Work out the finished part from the listing and answer in its coordinate system (mm). Round coordinates to 2 decimals unless told otherwise and drop trailing zeros. Order: outer loops, then holes, each group sorted by start corner. A loop starts at its lowest first (then second) coordinate and runs counter-clockwise, first axis right, second up. Notation, with made-up numbers: (29, -20.75) -> (68, -20.75) arc R16 cw to (68, -9.75) -> close; hole circle Ø10 at (12, -13.75). An arc over 180 degrees is marked (long way). Use a Markdown table: item, result. Add a question column.
Item 1: Find the intervals of material crossed by L1, parallel to Z at x = 37, y = 3; L2, parallel to Z at x = 35, y = 2.6; L3, parallel to X at y = 1.1, z = 9, in increasing order. Write a range as [from, to].
Item 2: A cutting plane is placed at B-B, the plane y = 1.7. Give the number of separate pieces and of enclosed holes in the cut face, plus the area to 3 significant figures.
Item 3: A cutting plane is placed at C-C, the plane x = 57.5. Determine the outline of the cut face in (y, z).
Item 4: A cutting plane is placed at A-A, the plane x = 0. Determine the outline of the cut face in (y, z).
Item 5: Flat-ended cylindrical pins translate along their axes: P1, Ø4.5, axis at x = 5, z = 0, coming from the +Y side; P2, Ø1, axis at y = 3.5, z = 6.5, coming from the +X side. Find the tip coordinate at first contact, or state that the pin passes through.
from build123d import *

# Parameters (mm, degrees)
SKETCH_1_R      = 1.35
SKETCH_1_R_2    = 1.5
SKETCH_1_R_3    = 7.1
EXTRUDE_1_DEPTH = 5
SKETCH_1_3_R    = 7.1
SKETCH_1_3_R_2  = 3.5
EXTRUDE_2_DEPTH = 3
FILLET_1_R      = 1
CHAMFER_1_SIZE  = 0.6
CHAMFER_2_SIZE  = 1


with BuildPart() as part:
    # Sketch 1 → Extrude 1 (new body)
    with BuildSketch(Plane(origin=(0, 0, 0), x_dir=(1, 0, 0), z_dir=(0, 1, 0))):
        with BuildLine():
            Line((1.6, -15.919798994), (61, -9.949874371))
            ThreePointArc((61, -9.949874371), (70, 0), (61, 9.949874371))
            Line((61, 9.949874371), (1.6, 15.919798994))
            ThreePointArc((1.6, 15.919798994), (-16, 0), (1.6, -15.919798994))
        make_face()
        with Locations(Location((-5, 0, 0), (0, 0, 270))):
            Circle(SKETCH_1_R, mode=Mode.SUBTRACT)
        with Locations(Location((0, 5, 0), (0, 0, 270))):
            Circle(SKETCH_1_R, mode=Mode.SUBTRACT)
        with Locations(Location((5, 0, 0), (0, 0, 270))):
            Circle(SKETCH_1_R, mode=Mode.SUBTRACT)
        with Locations(Location((0, -5, 0), (0, 0, 270))):
            Circle(SKETCH_1_R, mode=Mode.SUBTRACT)
        with Locations(Location((0, 0, 0), (0, 0, 270))):
            Circle(SKETCH_1_R_2, mode=Mode.SUBTRACT)
        with Locations(Location((60, 0, 0), (0, 0, 270))):
            Circle(SKETCH_1_R_3, mode=Mode.SUBTRACT)
        Polygon((19.888927579, 9.056503536), (47.567517096, 6.274700622), (37.219953316, 2.152836244), align=None, mode=Mode.SUBTRACT)
        Polygon((19.888927579, -9.056503536), (47.567517096, -6.274700622), (37.219953316, -2.152836244), align=None, mode=Mode.SUBTRACT)
        with BuildLine():
            Line((14.422056339, 6.928512895), (31.815454695, 0))
            Line((31.815454695, 0), (14.422056339, -6.928512895))
            ThreePointArc((14.422056339, -6.928512895), (16, 0), (14.422056339, 6.928512895))
        make_face(mode=Mode.SUBTRACT)
        with BuildLine():
            Line((42.624451937, 0), (50.505563121, -3.139373879))
            ThreePointArc((50.505563121, -3.139373879), (50, 0), (50.505563121, 3.139373879))
            Line((50.505563121, 3.139373879), (42.624451937, 0))
        make_face(mode=Mode.SUBTRACT)
        with BuildLine():
            ThreePointArc((6.268918397, -10.814372942), (8.838834765, -8.838834765), (10.814372942, -6.268918397))
            ThreePointArc((10.814372942, -6.268918397), (10.268918397, -4.218923436), (8.218923436, -4.764377982))
            ThreePointArc((8.218923436, -4.764377982), (6.717514421, -6.717514421), (4.764377982, -8.218923436))
            ThreePointArc((4.764377982, -8.218923436), (4.218923436, -10.268918397), (6.268918397, -10.814372942))
        make_face(mode=Mode.SUBTRACT)
        with BuildLine():
            ThreePointArc((-10.814372942, -6.268918397), (-8.838834765, -8.838834765), (-6.268918397, -10.814372942))
            ThreePointArc((-6.268918397, -10.814372942), (-4.218923436, -10.268918397), (-4.764377982, -8.218923436))
            ThreePointArc((-4.764377982, -8.218923436), (-6.717514421, -6.717514421), (-8.218923436, -4.764377982))
            ThreePointArc((-8.218923436, -4.764377982), (-10.268918397, -4.218923436), (-10.814372942, -6.268918397))
        make_face(mode=Mode.SUBTRACT)
        with BuildLine():
            ThreePointArc((-6.268918397, 10.814372942), (-8.838834765, 8.838834765), (-10.814372942, 6.268918397))
            ThreePointArc((-10.814372942, 6.268918397), (-10.268918397, 4.218923436), (-8.218923436, 4.764377982))
            ThreePointArc((-8.218923436, 4.764377982), (-6.717514421, 6.717514421), (-4.764377982, 8.218923436))
            ThreePointArc((-4.764377982, 8.218923436), (-4.218923436, 10.268918397), (-6.268918397, 10.814372942))
        make_face(mode=Mode.SUBTRACT)
        with BuildLine():
            ThreePointArc((10.814372942, 6.268918397), (8.838834765, 8.838834765), (6.268918397, 10.814372942))
            ThreePointArc((6.268918397, 10.814372942), (4.218923436, 10.268918397), (4.764377982, 8.218923436))
            ThreePointArc((4.764377982, 8.218923436), (6.717514421, 6.717514421), (8.218923436, 4.764377982))
            ThreePointArc((8.218923436, 4.764377982), (10.268918397, 4.218923436), (10.814372942, 6.268918397))
        make_face(mode=Mode.SUBTRACT)
    extrude(amount=EXTRUDE_1_DEPTH)

    # Sketch 1_3 → Extrude 2 (add)
    with BuildSketch(Plane(origin=(0, 0, 0), x_dir=(1, 0, 0), z_dir=(0, 1, 0))):
        with Locations(Location((60, 0, 0), (0, 0, 270))):
            Circle(SKETCH_1_3_R)
        with Locations(Location((60, 0, 0), (0, 0, 270))):
            Circle(SKETCH_1_3_R_2, mode=Mode.SUBTRACT)
    extrude(amount=EXTRUDE_2_DEPTH)

    # Fillet 1
    fillet_1_edges = [part.edges().sort_by_distance(p)[0] for p in [
        (47.567517096, 2.5, -6.274700622),
        (19.888927579, 2.5, -9.056503536),
        (37.219953316, 2.5, -2.152836244),
        (19.888927579, 2.5, 9.056503536),
        (47.567517096, 2.5, 6.274700622),
        (37.219953316, 2.5, 2.152836244),
        (42.624451937, 2.5, 0),
        (50.505563121, 2.5, 3.139373879),
        (50.505563121, 2.5, -3.139373879),
        (31.815454695, 2.5, 0),
        (14.422056339, 2.5, -6.928512895),
        (14.422056339, 2.5, 6.928512895),
    ]]
    fillet(fillet_1_edges, radius=FILLET_1_R)

    # Chamfer 1
    chamfer_1_edges = [part.edges().sort_by_distance(p)[0] for p in [
        (31.3, 5, 12.934836682),
        (70, 5, 0),
        (31.3, 5, -12.934836682),
        (-16, 5, 0),
        (-16, 0, 0),
        (31.3, 0, -12.934836682),
        (70, 0, 0),
        (31.3, 0, 12.934836682),
    ]]
    chamfer(chamfer_1_edges, length=CHAMFER_1_SIZE)

    # Chamfer 2
    chamfer_2_edges = [part.edges().sort_by_distance(p)[0] for p in [
        (-5, 5, -1.35),
        (0, 5, -6.35),
        (5, 5, -1.35),
        (0, 5, 3.65),
    ]]
    chamfer(chamfer_2_edges, length=CHAMFER_2_SIZE)


solid = part.part
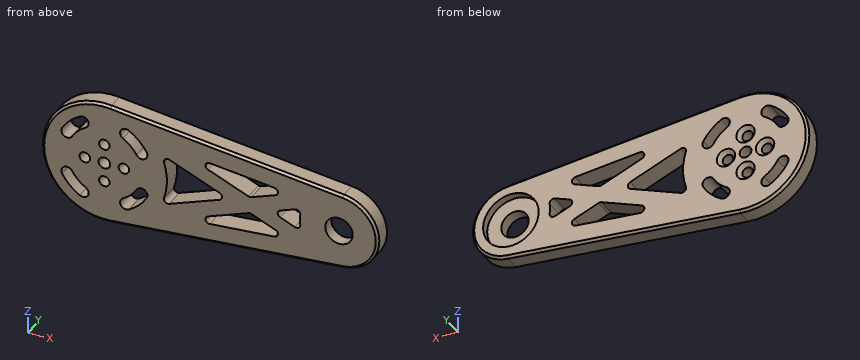
Reported:
| question | item | result |
|---|---|---|
| 1 | L1 | [-12.36, -7.34], [-2.25, 2.25], [7.34, 12.36] |
| 1 | L2 | [-12.56, -7.54], [-3.04, 3.04], [7.54, 12.56] |
| 1 | L3 | [-13.23, -8.67], [-4.11, 4.11], [8.67, 64.36] |
| 2 | separate pieces | 1 |
| 2 | enclosed holes | 14 |
| 2 | area | 1,710 mm² |
| 3 | outline | (0, -9.7) -> (0.6, -10.3) -> (4.4, -10.3) -> (5, -9.7) -> (5, -6.65) -> (3, -6.65) -> (3, -2.45) -> (0, -2.45) -> close; (0, 2.45) -> (3, 2.45) -> (3, 6.65) -> (5, 6.65) -> (5, 9.7) -> (4.4, 10.3) -> (0.6, 10.3) -> (0, 9.7) -> close |
| 4 | outline | (0, -15.4) -> (0.6, -16) -> (4.4, -16) -> (5, -15.4) -> (5, -7.35) -> (4, -6.35) -> (0, -6.35) -> close; (0, -3.65) -> (4, -3.65) -> (5, -2.65) -> (5, -1.5) -> (0, -1.5) -> close; (0, 1.5) -> (5, 1.5) -> (5, 2.65) -> (4, 3.65) -> (0, 3.65) -> close; (0, 6.35) -> (4, 6.35) -> (5, 7.35) -> (5, 15.4) -> (4.4, 16) -> (0.6, 16) -> (0, 15.4) -> close |
| 5 | P1 | y = 4.9 |
| 5 | P2 | x = 68 |
